Design review of the part shown in the three views and the two pictorial views. Dimensions are in mm from the part's minimum x, y and z. Coordinates: 2 decimals unless noted, no trailing zeros. Order: outer loops, then holes, each group sorted by start corner. A loop starts at its lowest first (then second) coordinate and runs counter-clockwise, first axis right, second up. Notation, with made-up numbers: (33, 33) - (44, 33) arc R32 cw to (44, 59) - close; hole circle Ø4 at (-25.5, 39). An arc over 180 degrees is marked (long way). One line per item, written item: value. Start each with the question number.
(1) Consider section A-A on x = 30. Write out the cut boundary in (y, z).
(2) To check wall thickness, follow line 1 along X through (y, z) = (66.5, 3.5) (1 decimal); line 2 along X through (y, z) = (30, 4) (1 decimal); line 3 along X through (y, z) = (106, 3.5) (1 decimal). State the ranges of each line that lie inside material, in increasing order.
(3) Consider section B-B on z = 1.75. Write out the cut boundary in (x, y) (1 decimal), then the cut area to 3 significant figures.
(4) Consider section D-D on y = 60. Write out the cut boundary in (x, z).
(5) Consider section C-C on y = 26.5. Write out the cut boundary in (x, z) (1 decimal).
(6) Mouldability with a two-part tool opening along Y and no side actions: class the marked faces 1, 2 and 3 as released by +Y, released by -Y, zero draft, split by the parting line, or undercut.
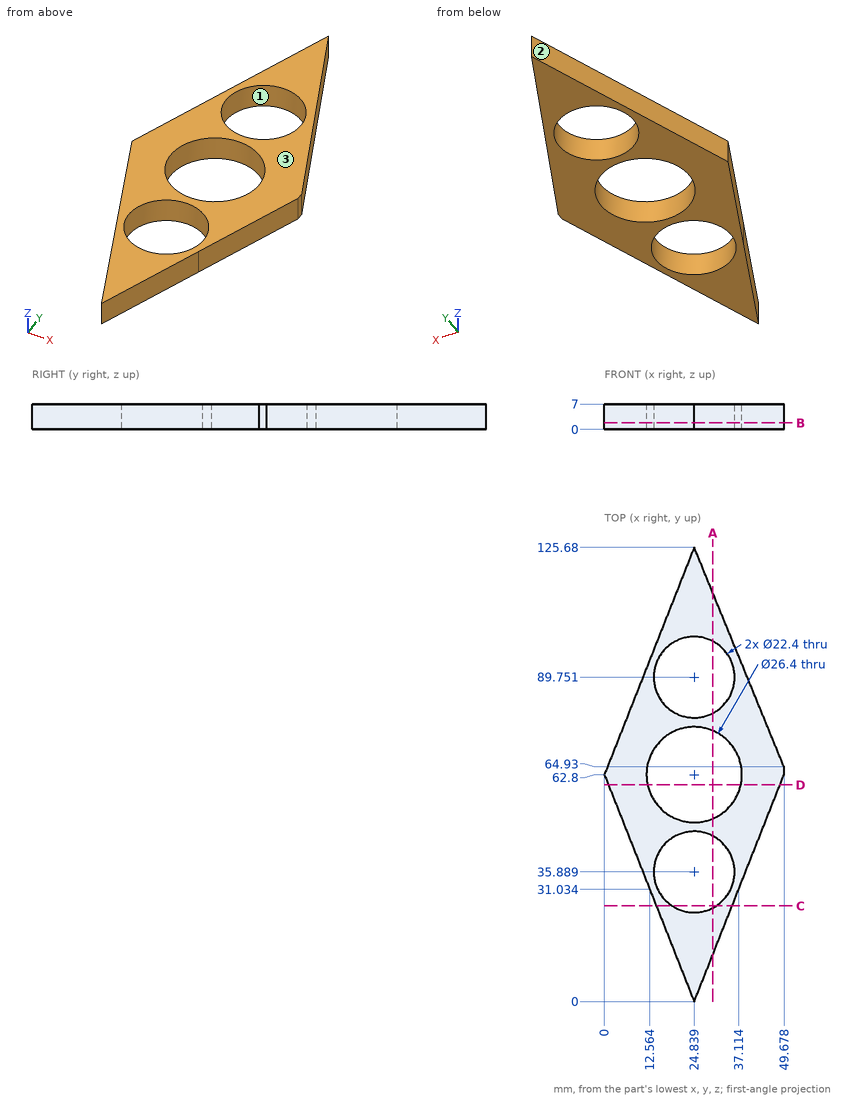
Geometry check:
1. outline: (13.05, 0) - (25.95, 0) - (25.95, 7) - (13.05, 7) - close; (45.83, 0) - (50.65, 0) - (50.65, 7) - (45.83, 7) - close; (74.95, 0) - (79.81, 0) - (79.81, 7) - (74.95, 7) - close; (99.69, 0) - (113.06, 0) - (113.06, 7) - (99.69, 7) - close
2. line 1: x = 1.5 to 12.2, 37.5 to 49
2. line 2: x = 13 to 15.3, 34.4 to 36.7
2. line 3: x = 17.1 to 32.9
3. outline: (0, 62.8) - (24.8, 0) - (49.7, 62.8) - (49.7, 64.9) - (24.8, 125.7) - close; hole circle Ø26.4 at (24.8, 62.8); hole circle Ø22.4 at (24.8, 35.9); hole circle Ø22.4 at (24.8, 89.8)
3. area: 1,810 mm^2
4. outline: (1.11, 0) - (11.94, 0) - (11.94, 7) - (1.11, 7) - close; (37.74, 0) - (48.57, 0) - (48.57, 7) - (37.74, 7) - close
5. outline: (14.4, 0) - (18.7, 0) - (18.7, 7) - (14.4, 7) - close; (30.9, 0) - (35.3, 0) - (35.3, 7) - (30.9, 7) - close
6. face 1: undercut
6. face 2: released by +Y
6. face 3: zero draft
